Geometry: final body of the model. Coordinates: model frame, mm. Round coordinates to 2 decimals unless told otherwise and drop trailing zeros. Write each loop counter-clockwise with the first axis right and the second up, starting at its lowest first coordinate (ties: lowest second). Pieces come first, ordered by that corner, then holes. Notation, with made-up numbers: M 63,16 L 70,16 A25 ccw 70,29 Z; hole C -8,38.5 d6. An arc over 180 degrees is marked long. Answer as CSV lines item,"result". Start each with the question number.
Q1. Section query B-B on z = 8. Output: boundary loops of the cut face in (x, y), and give its area (3 significant figures).
Q2. Ray query, probe 1 along Z at (x, y) = (-2.5, 4.5); probe 2 along Z at (x, y) = (-4.25, -8.25); probe 3 along X at (y, z) = (1.75, 10.5). Return the intervals inside material, ascending.
Q3. First-contact query: pin 1 (1.5 mm diameter, centred on y = 3.5, z = 10, fed in from +X); pin 2 (3 mm diameter, centred on x = -4, y = 5, fed in from +Z); pin 3 (1 mm diameter, centred on y = -1, z = 14, fed in from -X). Flat tips, straight axial feed; report the tip coordinate or a pass-through.
Q4. Section query A-A on z = 17. Output: boundary loops of the cut face in (x, y).
```python
from build123d import *

# Parameters (mm, degrees)
F0_R       = 10
F1_DEPTH   = 20
F2_SIZE2   = 5
F2_SIZE    = 4
F2_2_SIZE2 = 5
F2_2_SIZE  = 4
F3_R       = 5


with BuildPart() as f1:
    # F0 (on Top) → F1 (new body)
    with BuildSketch(Plane.XY):
        Circle(F0_R)
    extrude(amount=F1_DEPTH)

    # F2
    f2_edges = [f1.edges().sort_by_distance(p)[0] for p in [
        (-10, 0, 20),
    ]]
    f2_side = f1.faces().sort_by_distance((0, 0, 20))[0]
    chamfer(f2_edges, length=F2_SIZE, length2=F2_SIZE2, reference=f2_side)

    # F2#2
    f2_2_edges = [f1.edges().sort_by_distance(p)[0] for p in [
        (-10, 0, 0),
    ]]
    f2_2_side = f1.faces().sort_by_distance((0, 0, 0))[0]
    chamfer(f2_2_edges, length=F2_2_SIZE, length2=F2_2_SIZE2, reference=f2_2_side)

    # F3
    f3_edges = [f1.edges().sort_by_distance(p)[0] for p in [
        (-10, 0, 15),
        (-6, 0, 20),
        (-10, 0, 5),
    ]]
    fillet(f3_edges, radius=F3_R)


solid = f1.part
```
Entries:
1,outline,"C 0,0 d20"
1,area,"314 mm^2"
2,probe 1,"z = 0 to 19.75"
2,probe 2,"z = 4.17 to 15.83"
2,probe 3,"x = -9.85 to 9.85"
3,pin 1,"stops at x = 9.61"
3,pin 2,"stops at z = 19.83"
3,pin 3,"stops at x = -9.96"
4,outline,"C 0,0 d16.8"
